Part model, mm, in its own coordinate system. A direction names the side the tool comes from. Round coordinates to 2 decimals unless told otherwise and drop trailing zeros. Write each loop counter-clockwise with the first axis right and the second up, starting at its lowest first coordinate (ties: lowest second). Pieces come first, ordered by that corner, then holes. Notation, with made-up numbers: M 60,70.5 L 101,70.5 A16 cw 101,96.5 Z; hole C -25.75,-16 d6. An arc over 180 degrees is marked long. Answer as a JSON object with one key per item and string values. Group by question number.
1. Band-saw the part on B-B, the plane z = 0. Write the cut outline in (x, y), plus the area to 3 significant figures.
2. Band-saw the part on A-A, the plane x = 0. Write the cut outline in (y, z), plus the area to 3 significant figures.
3. Drop flat-ended pins along their axis: pin 1 (2 mm diameter, centred on y = 3, z = -6, fed in from +X); pin 2 (4 mm diameter, centred on y = 3.5, z = 12.5, fed in from -X); pin 3 (6.5 mm diameter, centred on x = 0, z = 18, fed in from +Y). Give the stop position or say it passes through.
4. Two-plate mould, pull along X, no slides. Class faces 3 (the face through (-3.62, 2.028, 22.996)), 4 (the face through (9.108, 2.028, -8.747)), 5 (the face through (-0.33, 1.97, -20.48)): +X half, -X half, draft (parallel to the pull), parting line (faces both ways), or undercut.
5. Which spindle directions (+Z, -Z, +X, -X, +Y, -Y) get a long thin tool onto all of the face, cutting with end or side? Do faces 1 (the face through (3, 4, -6)), 2 (the face through (-3.62, 2.028, -22.996)). Say none if no direction does.
6. Band-saw the part on C-C, the plane z = 5. Write the cut outline in (x, y), plus the area to 3 significant figures.
7. Drill centre lines: line 1 (Z direction, x = 0, y = 2.1); line 2 (X direction, y = 5, z = 0); line 3 (Y direction, x = -3.25, z = 9.5). Where is each one in solid material? Low to high. Write a range as from..to.
8. Band-saw the part on D-D, the plane z = -18. Write the cut outline in (x, y).
from build123d import *

# Parameters (mm, degrees)
SKETCH_1_R      = 2.5
SKETCH_1_R_2    = 12.5
SKETCH_1_R_3    = 4
EXTRUDE_1_DEPTH = 4
FILLET_1_R      = 5
SKETCH_2_R      = 6
SKETCH_2_R_2    = 4
EXTRUDE_2_DEPTH = 3


with BuildPart() as part:
    # 草图1 → 凸台-拉伸1 (new body)
    with BuildSketch(Plane(origin=(0, 0, 0), x_dir=(1, 0, 0), z_dir=(0, 1, 0))):
        with BuildLine():
            Line((-9.042322889, -8.630550201), (-4.305971765, -24))
            Line((-4.305971765, -24), (4.305971765, -24))
            Line((4.305971765, -24), (9.042322889, -8.630550201))
            ThreePointArc((9.042322889, -8.630550201), (0, -12.5), (-9.042322889, -8.630550201))
        make_face()
        with Locations((0, -18)):
            Circle(SKETCH_1_R, mode=Mode.SUBTRACT)
        Circle(SKETCH_1_R_2)
        Circle(SKETCH_1_R_3, mode=Mode.SUBTRACT)
        with BuildLine():
            Line((-4.305971765, 24), (-9.042322889, 8.630550201))
            ThreePointArc((-9.042322889, 8.630550201), (0, 12.5), (9.042322889, 8.630550201))
            Line((9.042322889, 8.630550201), (4.305971765, 24))
            Line((4.305971765, 24), (-4.305971765, 24))
        make_face()
        with Locations((0, 18)):
            Circle(SKETCH_1_R, mode=Mode.SUBTRACT)
    extrude(amount=EXTRUDE_1_DEPTH)

    # 圆角1
    fillet_1_edges = [part.edges().sort_by_distance(p)[0] for p in [
        (4.305971765, 2, 24),
        (-4.305971765, 2, 24),
        (-9.042322889, 2, 8.630550201),
        (-9.042322889, 2, -8.630550201),
        (-4.305971765, 2, -24),
        (4.305971765, 2, -24),
        (9.042322889, 2, -8.630550201),
        (9.042322889, 2, 8.630550201),
    ]]
    fillet(fillet_1_edges, radius=FILLET_1_R)

    # 草图2 → 凸台-拉伸2 (add)
    with BuildSketch(Plane(origin=(0, 4, 0), x_dir=(1, 0, 0), z_dir=(0, 1, 0))):
        Circle(SKETCH_2_R)
        Circle(SKETCH_2_R_2, mode=Mode.SUBTRACT)
    extrude(amount=EXTRUDE_2_DEPTH)


solid = part.part
Worked answers:
{
 "1": {"outline": "M -12.5,0 L -4,0 L -4,7 L -6,7 L -6,4 L -12.5,4 Z; M 4,0 L 12.5,0 L 12.5,4 L 6,4 L 6,7 L 4,7 Z", "area": "80.0 mm^2"},
 "2": {"outline": "M 0,-24 L 4,-24 L 4,-20.5 L 0,-20.5 Z; M 0,-15.5 L 4,-15.5 L 4,-6 L 7,-6 L 7,-4 L 0,-4 Z; M 0,4 L 7,4 L 7,6 L 4,6 L 4,15.5 L 0,15.5 Z; M 0,20.5 L 4,20.5 L 4,24 L 0,24 Z", "area": "132 mm^2"},
 "3": {"pin 1": "stops at x = 11.46", "pin 2": "stops at x = -8.47", "pin 3": "stops at y = 4"},
 "4": {"face 3": "-X half", "face 4": "+X half", "face 5": "undercut"},
 "5": {"face 1": "+Y", "face 2": "-Z, -X, +Y, -Y"},
 "6": {"outline": "M -11.46,0 L 11.46,0 L 11.46,4 L 3.32,4 L 3.32,7 L -3.32,7 L -3.32,4 L -11.46,4 Z", "area": "112 mm^2"},
 "7": {"line 1": "z = -24..-20.5, -15.5..-4, 4..15.5, 20.5..24", "line 2": "x = -6..-4, 4..6", "line 3": "y = 0..4"},
 "8": {"outline": "M -6.15,0 L -2.5,0 L -2.5,4 L -6.15,4 Z; M 2.5,0 L 6.15,0 L 6.15,4 L 2.5,4 Z"}
}
